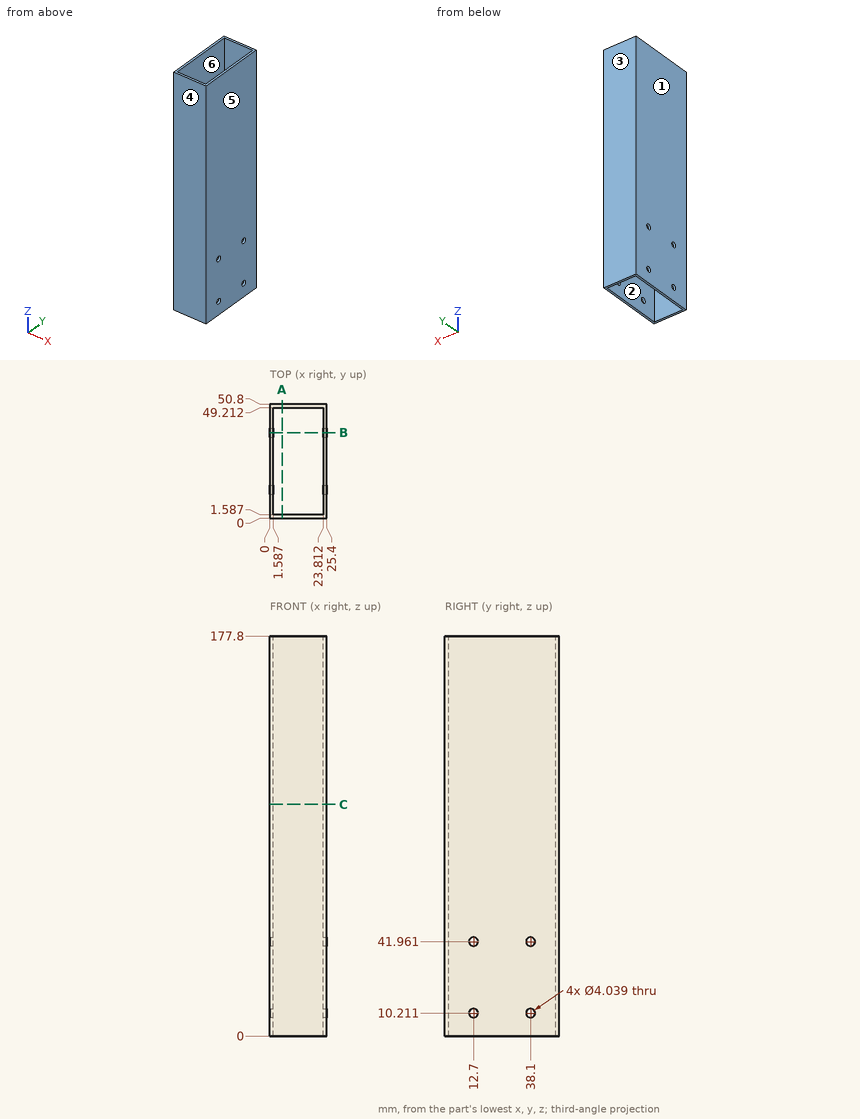
Part print with two shaded views. Sizes in mm from the minimum x, y, z corner. A direction names the side the tool comes from. Give positions to 0.01 mm unless a question says otherwise; leave off trailing zeros. Order: outer loops, then holes, each group sorted by start corner. A loop starts at its lowest first (then second) coordinate and runs counter-clockwise, first axis right, second up. Notation, with made-up numbers: (67.25, 84.5) - (125.25, 84.5) arc R21 ccw to (125.25, 107.5) - close; hole circle Ø1 at (55, -24). An arc over 180 degrees is marked (long way). Write each question's results on one line, items separated by ' | '.
1. Probe L1, parallel to Y at x = 14.25, z = 81; L2, parallel to X at y = 11, z = 83. List the from-to ranges inside material, lowest first. Write a range as from..to.
Calculated:
L1: y = 0..1.59, 49.21..50.8 | L2: x = 0..1.59, 23.81..25.4
2. Saw through at B-B on y = 38.1. List the corners of the cut face in (x, z).
Calculated:
outline: (0, 0) - (1.59, 0) - (1.59, 8.19) - (0, 8.19) - close; (0, 12.23) - (1.59, 12.23) - (1.59, 39.94) - (0, 39.94) - close; (0, 43.98) - (1.59, 43.98) - (1.59, 177.8) - (0, 177.8) - close; (23.81, 0) - (25.4, 0) - (25.4, 8.19) - (23.81, 8.19) - close; (23.81, 12.23) - (25.4, 12.23) - (25.4, 39.94) - (23.81, 39.94) - close; (23.81, 43.98) - (25.4, 43.98) - (25.4, 177.8) - (23.81, 177.8) - close
3. 3-axis set-ups, long thin cutter, end or side, ignore diameter. For the marked faces 5 and 6: which of +Z, -Z, +X, -X, +Y, -Y reach the whole face in a straight line?
Calculated:
face 5: +Z, -Z, +X, +Y, -Y | face 6: +Z, -Z
4. Pin check, flat tip, straight feed: pin 1 (3 mm diameter, centred on y = 12.7, z = 10.21, fed in from -X). Stop position of the tip, or through.
Calculated:
pin 1: passes through
5. Saw through at A-A on x = 5.5. List the corners of the cut face in (y, z).
Calculated:
outline: (0, 0) - (1.59, 0) - (1.59, 177.8) - (0, 177.8) - close; (49.21, 0) - (50.8, 0) - (50.8, 177.8) - (49.21, 177.8) - close
6. Pull direction Y, two halves, no side cores. Call the marked faces 1, 2, 3 and 4: released by +Y, released by -Y, zero draft, split by the parting line, or undercut.
Calculated:
face 1: zero draft | face 2: undercut | face 3: released by +Y | face 4: released by -Y
7. Saw through at C-C on z = 103. List the corners of the cut face in (x, y).
Calculated:
outline: (0, 0) - (25.4, 0) - (25.4, 50.8) - (0, 50.8) - close; hole (1.59, 1.59) - (23.81, 1.59) - (23.81, 49.21) - (1.59, 49.21) - close
